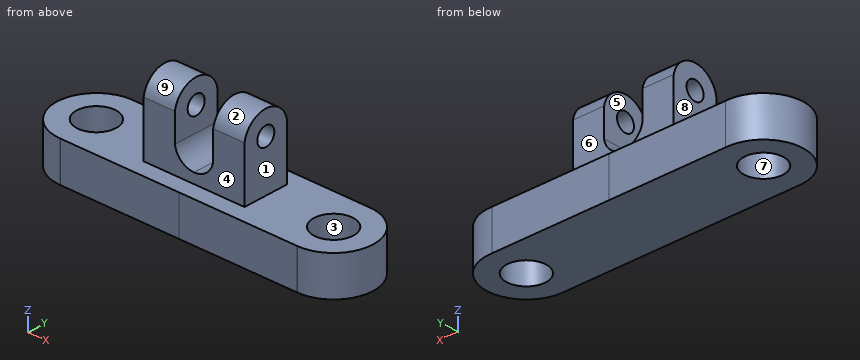
```python
from build123d import *

# Parameters (mm, degrees)
F0_R     = 6.35
F1_DEPTH = 12.7
F0_W     = 16.3278355569
F0_H     = 14.9416262284
F2_DEPTH = 38.1
F4_DEPTH = 25.4
F6_DEPTH = 25.4
F5_R     = 2.9883408706
F7_DEPTH = 25.4


with BuildPart() as f1:
    # F0 (on Top) → F1 (new body)
    with BuildSketch(Plane.XY):
        with BuildLine():
            Line((0.3017354131, 12.6927690867), (-37.4940995503, 12.6855384058))
            ThreePointArc((-37.4940995503, 12.6855384058), (-50.7954163284, 0.341180667), (-38.1763124432, -12.6997707228))
            Line((-38.1763124432, -12.6997707228), (-38.0237639047, -12.6997711813))
            Line((-38.0237639047, -12.6997711813), (0.3017354131, -12.6998863831))
            Line((0.3017354131, -12.6998863831), (0.3017354131, -7.3503162712))
            Line((0.3017354131, -7.3503162712), (-16.0261001438, -7.3503162712))
            Line((-16.0261001438, -7.3503162712), (-16.0261001438, 7.5913099572))
            Line((-16.0261001438, 7.5913099572), (0.3017354131, 7.5913099572))
            Line((0.3017354131, 7.5913099572), (0.3017354131, 12.6927690867))
        make_face()
        with Locations((-38.1, 0)):
            Circle(F0_R, mode=Mode.SUBTRACT)
    extrude(amount=F1_DEPTH)

    # F0 (on Top) → F2 (join)
    with BuildSketch(Plane.XY):
        with Locations((-7.8621823653, 0.120496843)):
            Rectangle(F0_W, F0_H)
    extrude(amount=F2_DEPTH)

    # F3 (on face) → F4 (cut)
    with BuildSketch(Plane.XZ.offset(7.3503162712)):
        with BuildLine():
            Line((-5.9043527581, 38.1), (-5.9043527581, 21.2074704468))
            ThreePointArc((-5.9043527581, 21.2074704468), (-3.7853007654, 17.4047273656), (0.3017354131, 15.9056037664))
            Line((0.3017354131, 15.9056037664), (0.3017354131, 38.1))
            Line((0.3017354131, 38.1), (-5.9043527581, 38.1))
        make_face()
    extrude(amount=-F4_DEPTH, mode=Mode.SUBTRACT)

    # F5 (on face) → F6 (cut)
    with BuildSketch(Plane(origin=(-16.0261001438, 0, 0), x_dir=(0, -1, 0), z_dir=(-1, 0, 0))):
        with BuildLine():
            ThreePointArc((-7.5913099572, 30.2173364908), (-0.120496843, 36.4995504426), (7.3503162712, 30.2173364908))
            Line((7.3503162712, 30.2173364908), (7.3503162712, 38.1))
            Line((7.3503162712, 38.1), (-7.5913099572, 38.1))
            Line((-7.5913099572, 38.1), (-7.5913099572, 30.2173364908))
        make_face()
    extrude(amount=-F6_DEPTH, mode=Mode.SUBTRACT)

    # F5 (on face) → F7 (cut)
    with BuildSketch(Plane(origin=(-16.0261001438, 0, 0), x_dir=(0, -1, 0), z_dir=(-1, 0, 0))):
        with Locations((-0.120496843, 28.9162954426)):
            Circle(F5_R)
    extrude(amount=-F7_DEPTH, mode=Mode.SUBTRACT)

    # F8: F1 across face


with BuildPart() as f1_1:
    add(f1.part)
    add(f1.part.mirror(Plane(origin=(0.3017354131, 0.0124838458, 7.3784331219), x_dir=(0, 1, 0), z_dir=(1, 0, 0))))


solid = f1_1.part
```
Verification items for the finished model (mm, model axes). Face numbers are marked on the shaded views. A direction names the side the tool comes from. Round coordinates to 2 decimals unless told otherwise and drop trailing zeros. Write each loop counter-clockwise with the first axis right and the second up, starting at its lowest first coordinate (ties: lowest second). Pieces come first, ordered by that corner, then holes. Notation, with made-up numbers: (80, 78.25) - (112, 78.25) arc R32 ccw to (112, 112.25) - close; hole circle Ø5 at (18, 13). An arc over 180 degrees is marked (long way). Answer as a JSON object with one key per item and string values. Group by question number.
Q1. Section check D-D, the plane x = 35.5. Enter the section's corners in (y, z), plus the area to 3 significant figures.
Q2. Go/stop test with flat-tipped pins: pin 1 Ø4 at (x, z) = (-17, 3) entering from +Y; pin 2 Ø12.5 at (x, y) = (-8, -5.5) entering from +Z; pin 3 Ø5.5 at (x, z) = (7, 20) entering from -Y; pin 4 Ø3 at (y, z) = (4, 6.5) entering from -X. Record where each tip stops, or that it passes through.
Q3. Mould release check, pull along Y, two halves, no side actions. Record for the marked faces 1, 2, 3 and 4: released by +Y, released by -Y, zero draft, split by the parting line, or undercut.
Q4. Tool access check on the marked faces 5, 6, 7, 8 and 9. Record the directions out of +Z, -Z, +X, -X, +Y, -Y that give a thin tool (end or side, any length) a straight path to the whole face; none if there is none.
Q5. Thickness scan on line 1 (X direction, y = 0.5, z = 8); line 2 (X direction, y = 4, z = 34); line 3 (X direction, y = -4.75, z = 12.5). Record the ranges inside material, lowest first.
Q6. Section check C-C, the plane z = 23. Enter the section's corners in (x, y).
Q7. Section check B-B, the plane y = 0. Give the number of separate pieces and of enclosed holes in the cut face, plus the area to 3 significant figures.
Q8. Section check A-A, the plane z = 7. Enter the section's corners in (x, y).
Found:
{
 "1": {"outline": "(-12.7, 0) - (-5.48, 0) - (-5.48, 12.7) - (-12.7, 12.7) - close; (5.48, 0) - (12.69, 0) - (12.69, 12.7) - (5.48, 12.7) - close", "area": "183 mm^2"},
 "2": {"pin 1": "stops at y = 12.69", "pin 2": "stops at z = 36.5", "pin 3": "stops at y = -7.35", "pin 4": "stops at x = -50.55"},
 "3": {"face 1": "zero draft", "face 2": "split by the parting line", "face 3": "undercut", "face 4": "released by -Y"},
 "4": {"face 5": "+Z, +Y, -Y", "face 6": "+Z, +X, -X, +Y", "face 7": "+Z, -Z", "face 8": "+Z, -X, +Y, -Y", "face 9": "+Z, +X, -X"},
 "5": {"line 1": "x = -50.79 to -44.43, -31.77 to 32.37, 45.03 to 51.39", "line 2": "x = -16.03 to -5.9, 6.51 to 16.63", "line 3": "x = -49.88 to -42.31, -33.89 to 34.49, 42.92 to 50.48"},
 "6": {"outline": "(-16.03, -7.35) - (-5.9, -7.35) - (-5.9, 7.59) - (-16.03, 7.59) - close; (6.51, -7.35) - (16.63, -7.35) - (16.63, 7.59) - (6.51, 7.59) - close"},
 "7": {"separate pieces": "5", "enclosed holes": "0", "area": "1,390 mm^2"},
 "8": {"outline": "(-38.18, -12.7) - (0.3, -12.7) - (38.78, -12.7) arc R12.7 ccw (long way) to (38.1, 12.69) - (0.3, 12.69) - (-37.49, 12.69) arc R12.7 ccw (long way) to start; hole circle Ø12.7 at (-38.1, 0); hole circle Ø12.7 at (38.7, 0)"}
}
